```python
from build123d import *
from OCP.BRepFilletAPI import BRepFilletAPI_MakeChamfer

# Parameters (mm, degrees)
BOSS_EXTRUDE1_DEPTH        = 4
BOSS_EXTRUDE2_DEPTH        = 64
SKETCH3_W                  = 35
SKETCH3_H                  = 51
CUT_EXTRUDE1_DEPTH         = 101.369318021
CUT_EXTRUDE2_DEPTH         = 123.474487139
CHAMFER1_SIZE              = 10
CHAMFER1_SIZE2             = 8.390996312
F_4_5_4_5_DIAMETER_HOLE1_D = 4.5
CUT_EXTRUDE3_DEPTH         = 109.166538264
CUT_EXTRUDE4_DEPTH         = 111.113577728
CUT_EXTRUDE5_DEPTH         = 10
CHAMFER3_SIZE              = 2


with BuildPart() as part:
    # Sketch1 → Boss-Extrude1 (new body)
    with BuildSketch(Plane(origin=(0, 0, 0), x_dir=(1, 0, 0), z_dir=(0, 1, 0))):
        Polygon((-35, 29), (0, 74), (6, 74), (35, 29), (35, -29), (-35, -29), align=None)
    extrude(amount=BOSS_EXTRUDE1_DEPTH)

    # Sketch2 → Boss-Extrude2 (add)
    with BuildSketch(Plane(origin=(0, 4, 0), x_dir=(1, 0, 0), z_dir=(0, 1, 0))):
        Polygon((35, 29), (21.75, 29), (0, 9), (-18, 9), (-18, 18.5), (-35, 18.5), (-35, 29), (0, 74), (6, 74), align=None)
    extrude(amount=BOSS_EXTRUDE2_DEPTH)

    # Sketch3 → Cut-Extrude1 (cut, through all)
    with BuildSketch(Plane.XY.offset(-9)):
        Polygon((-35, 4), (-10, 68), (-35, 68), align=None)
        with Locations((17.5, 42.5)):
            Rectangle(SKETCH3_W, SKETCH3_H)
    extrude(amount=-CUT_EXTRUDE1_DEPTH, mode=Mode.SUBTRACT)

    # Sketch4 → Cut-Extrude2 (cut, through all)
    with BuildSketch(Plane(origin=(35, 0, 0), x_dir=(0, 0, -1), z_dir=(1, 0, 0))):
        Polygon((60, 0), (74, 20), (74, 0), align=None)
        Polygon((60, 68), (74, 68), (74, 48), align=None)
    extrude(amount=-CUT_EXTRUDE2_DEPTH, mode=Mode.SUBTRACT)

    # Chamfer1: one chamfer whose edges measure the first distance from different faces: ONE call of the kernel's chamfer builder (chamfer() names one face for all edges)
    chamfer1_edges_1 = [part.edges().sort_by_distance(p)[0] for p in [
        (-9, 4, -9),
    ]]
    chamfer1_side_1 = [part.faces().sort_by_distance(p)[0] for p in [
        (-8.515151515, 34.072854864, -9),
    ]]
    chamfer1_edges_2 = [part.edges().sort_by_distance(p)[0] for p in [
        (10.875, 4, -19),
    ]]
    chamfer1_side_2 = [part.faces().sort_by_distance(p)[0] for p in [
        (10.875, 10.5, -19),
    ]]
    chamfer1_edges_3 = [part.edges().sort_by_distance(p)[0] for p in [
        (28.375, 4, -29),
    ]]
    chamfer1_side_3 = [part.faces().sort_by_distance(p)[0] for p in [
        (28.375, 10.5, -29),
    ]]
    chamfer1 = BRepFilletAPI_MakeChamfer(part.part.solid().wrapped)
    for e in chamfer1_edges_1:
        chamfer1.Add(CHAMFER1_SIZE, CHAMFER1_SIZE2, e.wrapped, chamfer1_side_1[0].wrapped)  # the first distance lies on this face
    for e in chamfer1_edges_2:
        chamfer1.Add(CHAMFER1_SIZE, CHAMFER1_SIZE2, e.wrapped, chamfer1_side_2[0].wrapped)  # the first distance lies on this face
    for e in chamfer1_edges_3:
        chamfer1.Add(CHAMFER1_SIZE, CHAMFER1_SIZE2, e.wrapped, chamfer1_side_3[0].wrapped)  # the first distance lies on this face
    add(Compound.cast(chamfer1.Shape()), mode=Mode.REPLACE)

    # Ø4.5 (4.5) Diameter Hole1 (through all)
    with Locations(Plane(origin=(0, 0, 0), x_dir=(0, 0, -1), z_dir=(1, 0, 0))):
        with Locations((16.5, 44), (26.5, 31.5), (26.5, 56.5)):
            Hole(F_4_5_4_5_DIAMETER_HOLE1_D / 2)

    # Sketch9 → Cut-Extrude3 (cut, through all)
    with BuildSketch(Plane(origin=(-5, 0, 0), x_dir=(0, 0, -1), z_dir=(1, 0, 0))):
        Polygon((29.964101615, 56.5), (28.232050808, 59.5), (24.767949192, 59.5), (23.035898385, 56.5), (24.767949192, 53.5), (28.232050808, 53.5), align=None)
        Polygon((29.964101615, 31.5), (28.232050808, 34.5), (24.767949192, 34.5), (23.035898385, 31.5), (24.767949192, 28.5), (28.232050808, 28.5), align=None)
        Polygon((19.964101615, 44), (18.232050808, 47), (14.767949192, 47), (13.035898385, 44), (14.767949192, 41), (18.232050808, 41), align=None)
    extrude(amount=-CUT_EXTRUDE3_DEPTH, mode=Mode.SUBTRACT)

    # Sketch10 → Cut-Extrude4 (cut, through all)
    with BuildSketch(Plane(origin=(-10, 0, 0), x_dir=(0, 0, -1), z_dir=(1, 0, 0))):
        Polygon((30.887862046, 56.5), (28.693931023, 60.3), (24.306068977, 60.3), (22.112137954, 56.5), (24.306068977, 52.7), (28.693931023, 52.7), align=None)
        Polygon((20.887862046, 44), (18.693931023, 47.8), (14.306068977, 47.8), (12.112137954, 44), (14.306068977, 40.2), (18.693931023, 40.2), align=None)
        Polygon((30.887862046, 31.5), (28.693931023, 35.3), (24.306068977, 35.3), (22.112137954, 31.5), (24.306068977, 27.7), (28.693931023, 27.7), align=None)
    extrude(amount=-CUT_EXTRUDE4_DEPTH, mode=Mode.SUBTRACT)

    # Sketch11 → Cut-Extrude5 (cut)
    with BuildSketch(Plane(origin=(0, 4, 0), x_dir=(1, 0, 0), z_dir=(0, 1, 0))):
        with BuildLine():
            Line((-28.11, -17.6), (-23.11, -17.6))
            ThreePointArc((-23.11, -17.6), (-20.86, -19.85), (-23.11, -22.1))
            Line((-23.11, -22.1), (-28.11, -22.1))
            ThreePointArc((-28.11, -22.1), (-30.36, -19.85), (-28.11, -17.6))
        make_face()
        with BuildLine():
            Line((24.09, -17.6), (29.09, -17.6))
            ThreePointArc((29.09, -17.6), (31.34, -19.85), (29.09, -22.1))
            Line((29.09, -22.1), (24.09, -22.1))
            ThreePointArc((24.09, -22.1), (21.84, -19.85), (24.09, -17.6))
        make_face()
        with BuildLine():
            Line((-28.11, 14.9), (-23.11, 14.9))
            ThreePointArc((-23.11, 14.9), (-20.86, 12.65), (-23.11, 10.4))
            Line((-23.11, 10.4), (-28.11, 10.4))
            ThreePointArc((-28.11, 10.4), (-30.36, 12.65), (-28.11, 14.9))
        make_face()
        with BuildLine():
            Line((24.09, 14.9), (29.09, 14.9))
            ThreePointArc((29.09, 14.9), (31.34, 12.65), (29.09, 10.4))
            Line((29.09, 10.4), (24.09, 10.4))
            ThreePointArc((24.09, 10.4), (21.84, 12.65), (24.09, 14.9))
        make_face()
    extrude(amount=-CUT_EXTRUDE5_DEPTH, mode=Mode.SUBTRACT)

    # Chamfer3
    chamfer3_edges = [part.edges().sort_by_distance(p)[0] for p in [
        (21.84, 4, 19.85),
        (26.59, 4, 22.1),
        (31.34, 4, 19.85),
        (26.59, 4, 17.6),
        (-30.36, 4, -12.65),
        (-25.61, 4, -10.4),
        (-20.86, 4, -12.65),
        (-25.61, 4, -14.9),
        (21.84, 4, -12.65),
        (26.59, 4, -10.4),
        (31.34, 4, -12.65),
        (26.59, 4, -14.9),
        (-30.36, 4, 19.85),
        (-25.61, 4, 22.1),
        (-20.86, 4, 19.85),
        (-25.61, 4, 17.6),
    ]]
    chamfer(chamfer3_edges, length=CHAMFER3_SIZE)


solid = part.part
```
For this review, take the finished solid that the model builds, in its own axes (mm). A direction names the side the tool comes from. Give positions to 0.01 mm unless a question says otherwise; leave off trailing zeros. Write each loop counter-clockwise with the first axis right and the second up, starting at its lowest first coordinate (ties: lowest second). Pieces come first, ordered by that corner, then holes.
Item 1: Wall thickness on probe 1 along Y at (x, z) = (-3.25, -26.5); probe 2 along Z at (x, y) = (-1, 56); probe 3 along Y at (x, z) = (19, -36): over which ranges is each line inside the solid? List them lowest first.
Item 2: Take a section at C-C (x = 5). Give the boundary of the cut face in (y, z).
Item 3: Machinability: for faces 4 (the face through (21.84, 1.01, -12.6)), 5 (the face through (-7.5, 30, -23.9)), 6 (the face through (2.25, 7.64, -65.35)), which of the approach directions +Z, -Z, +X, -X, +Y, -Y give a long, thin tool a straight path to every point of the face, cutting with its end or side? Answer none if there is none.
Item 4: Insertion check: P1, Ø10, axis at y = 11.5, z = 12, coming from the -X side; P2, Ø10, axis at x = -25.5, y = 32, coming from the +Z side; P3, Ø17.5, axis at x = 11, z = -31, coming from the +Y side; P4, Ø6, axis at y = 56.5, z = -26, coming from the -X side. Each pin has a flat end and moves straight along its axis. Give the tip position at first contact, or say it passes through.
Item 5: Take a section at D-D (y = 63.5). Give the boundary of the cut face in (x, z).
Item 6: Take a section at A-A (z = -33.5). Give the boundary of the cut face in (x, y).
Item 7: The part is to be moulded in two halves that separate along Y. For faces 1 (the face through (-13.94, 42.13, -13.19)), 2 (the face through (31.34, 1.01, 19.8)), 3 (the face through (12.72, 8.93, -14.92)), say which applies: +Y half, -Y half, draft (parallel to the pull), parting line (faces both ways), or undercut.
Item 8: Take a section at B-B (x = -3). Give the boundary of the cut face in (y, z), and give its area (3 significant figures).
Established:
1. probe 1: y = 0 to 29.25, 33.75 to 54.25, 58.75 to 68
1. probe 2: z = -68.4 to -28.69, -24.31 to -9
1. probe 3: y = 0 to 17
2. outline: (0, -60) - (17, -71.9) - (17, -13.6) - (14, -13.6) - (4, -2.2) - (4, 29) - (0, 29) - close
3. face 4: +Y, -Y
3. face 5: -X
3. face 6: -Z, +X, -X, -Y
4. P1: passes through
4. P2: stops at z = -18.5
4. P3: stops at y = 17
4. P4: stops at x = -10
5. outline: (-11.76, -58.88) - (-8.44, -63.15) - (0, -63.15) - (0, -9) - (-11.76, -9) - close
6. outline: (-31.5, 0) - (32.1, 0) - (32.1, 17) - (0, 17) - (0, 68) - (-10, 68) - (-31.5, 12.96) - close
7. face 1: undercut
7. face 2: draft
7. face 3: +Y half
8. outline: (0, -60) - (14.49, -70.14) - (53.51, -70.14) - (68, -60) - (68, -9) - (14, -9) - (4, -0.61) - (4, 29) - (0, 29) - close; hole circle Ø4.5 at (31.5, -26.5); hole circle Ø4.5 at (44, -16.5); hole circle Ø4.5 at (56.5, -26.5)
8. area: 4,160 mm2
